Autodesk Inventor part; units mm, degrees
ref_plane "YZ Plane" through (0, 0, 0) normal (1, 0, 0) x (0, 1, 0)
ref_plane "XZ Plane" through (0, 0, 0) normal (0, 1, 0) x (-1, 0, 0)
ref_plane "XY Plane" through (0, 0, 0) normal (0, 0, 1) x (1, 0, 0)
sketch "スケッチ1" plane through (0, 0, 0) normal (0, 1, 0) x (-1, 0, 0)
  line L0 (7.5, -7.5) -> (-7.5, -7.5)
  line L1 (-7.5, -7.5) -> (-7.5, 7.5)
  line L2 (-7.5, 7.5) -> (7.5, 7.5)
  line L3 (7.5, 7.5) -> (7.5, -7.5)
  line L4 (7.5, -7.5) -> (-7.5, 7.5) construction
  line L5 (-7.5, -7.5) -> (7.5, 7.5) construction
  line L6 (6, -6) -> (-6, -6)
  line L7 (-6, -6) -> (-6, 6)
  line L8 (-6, 6) -> (6, 6)
  line L9 (6, 6) -> (6, -6)
  point P0 (0, 0)
  dimension "d0" = 15
  dimension "d1" = 15
  dimension "d2" = 1.5
extrude "押し出し1" add sketch "スケッチ1" along normal blind 88
sketch "スケッチ2" plane through (-7.5, 0, 7.5) normal (0, 0, 1) x (1, 0, 0)
  line L0 (7.5, 0) -> (7.5, 88) construction
  line L1 (0, 88) -> (15, 88)
  line L2 (0, 0) -> (0, 88)
  line L3 (0, 44) -> (15, 44) construction
  line L4 (15, 0) -> (15, 88)
sketch "スケッチ3" plane through (7.5, 0, 7.5) normal (1, 0, 0) x (0, 0, -1)
  line L0 (7.5, 0) -> (7.5, 88) construction
  line L1 (0, 88) -> (15, 88)
  line L2 (15, 0) -> (15, 88)
  line L3 (15, 44) -> (0, 44) construction
  line L4 (0, 0) -> (0, 88)
sketch "スケッチ4" plane through (-7.5, 0, 7.5) normal (0, 0, 1) x (1, 0, 0)
  line L0 (7.5, 0) -> (7.5, 88) construction
  circle A0 centre (7.5, 7.5) radius 1.5
  line L1 (0, 0) -> (15, 0)
  circle A1 centre (7.5, 68) radius 1.5
  line L2 (0, 88) -> (15, 88)
  dimension "d5" = 3
  dimension "d6" = 7.5
  dimension "d13" = 3
  dimension "d14" = 20
extrude "押し出し2" cut sketch "スケッチ4" against normal through all
sketch "スケッチ5" plane through (7.5, 0, 7.5) normal (1, 0, 0) x (0, 0, -1)
  circle A0 centre (7.5, 20) radius 1.5
  line L0 (7.5, 0) -> (7.5, 88) construction
  line L1 (0, 0) -> (15, 0)
  circle A1 centre (7.5, 80.5) radius 1.5
  line L2 (0, 88) -> (15, 88)
  dimension "d9" = 3
  dimension "d10" = 20
  dimension "d15" = 3
  dimension "d16" = 7.5
extrude "押し出し3" cut sketch "スケッチ5" against normal through all
sketch "スケッチ6" plane through (7.5, 0, 7.5) normal (1, 0, 0) x (0, 0, -1)
  circle A0 centre (7.5, 80.5) radius 1.5
  line L0 (0, 88) -> (15, 88)
  circle A1 centre (7.5, 20) radius 1.5
  line L1 (0, 0) -> (15, 0)
  point P0 (7.5, 0)
  dimension "d17" = 7.5
  dimension "d18" = 68
  dimension "d19" = 88
sketch "スケッチ7" plane through (-7.5, 0, 7.5) normal (0, 0, 1) x (1, 0, 0)
  circle A0 centre (7.5, 68) radius 1.5
  line L0 (0, 88) -> (15, 88)
  circle A1 centre (7.5, 7.5) radius 1.5
  point P0 (7.5, 0)
  dimension "d20" = 20
  dimension "d21" = 80.5
equation "\"d1\" = d0"
properties part number "omu_k_jo_11" material "アルミニウム 6061-AHC"
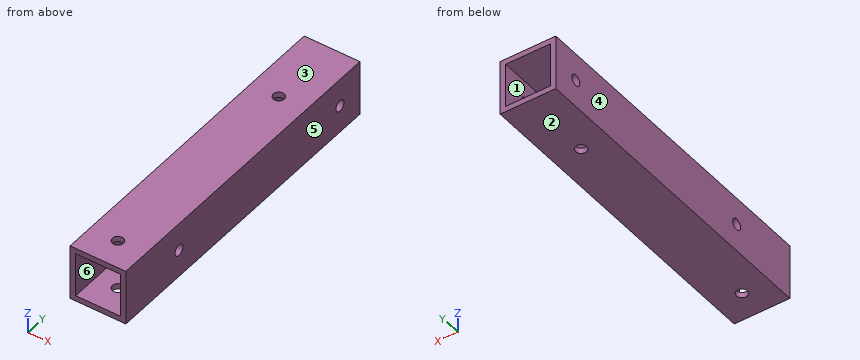
Design review of the part built by this model. Coordinates are the model's own, in mm. Face numbers are marked on the shaded views. A direction names the side the tool comes from. Round coordinates to 2 decimals unless told otherwise and drop trailing zeros. Write each loop counter-clockwise with the first axis right and the second up, starting at its lowest first coordinate (ties: lowest second). Pieces come first, ordered by that corner, then holes. Notation, with made-up numbers: (14, 51.5) - (61, 51.5) arc R16 ccw to (61, 63.5) - close; hole circle Ø1 at (-15, 24.25). An arc over 180 degrees is marked (long way). Return JSON: item names as keys, results as strings. Group by question number.
Item 1: We need section A-A on z = 0. Write out the cut boundary in (x, y).
Item 2: We need section C-C on y = 68. Write out the cut boundary in (x, z), and give its area (3 significant figures).
Item 3: Insertion check: P1, Ø2.5, axis at y = 80.5, z = 0, coming from the +X side. The pin has a flat end and moves straight along its axis. Give the tip position at first contact, or say it passes through.
Item 4: Machinability: for the marked faces 5 and 6, which of the approach directions +Z, -Z, +X, -X, +Y, -Y give a long, thin tool a straight path to every point of the face, cutting with its end or side? Answer none if there is none.
Item 5: The part is to be moulded in two halves that separate along Z. For the marked faces 1, 2, 3 and 4, say which applies: pulls with the +Z half, pulls with the -Z half, needs draft (parallel to the pull), parting line crosses it, or undercut.
Item 6: We need section D-D on x = -3.5. Write out the cut boundary in (y, z), and give its area (3 significant figures).
Item 7: For probe 1 along Y at (x, z) = (-6.4, 0); probe 2 along Z at (x, y) = (2.75, 51); probe 3 along Y at (x, z) = (0, -6.6), list the stretches that pass through material, from the lowest coordinate up. Write a range as [from, to].
Item 8: We need section B-B on x = 0. Write out the cut boundary in (y, z).
Model answer:
{
 "1": {"outline": "(-7.5, 0) - (-6, 0) - (-6, 18.5) - (-7.5, 18.5) - close; (-7.5, 21.5) - (-6, 21.5) - (-6, 79) - (-7.5, 79) - close; (-7.5, 82) - (-6, 82) - (-6, 88) - (-7.5, 88) - close; (6, 0) - (7.5, 0) - (7.5, 18.5) - (6, 18.5) - close; (6, 21.5) - (7.5, 21.5) - (7.5, 79) - (6, 79) - close; (6, 82) - (7.5, 82) - (7.5, 88) - (6, 88) - close"},
 "2": {"outline": "(-7.5, -7.5) - (-1.5, -7.5) - (-1.5, -6) - (-6, -6) - (-6, 6) - (-1.5, 6) - (-1.5, 7.5) - (-7.5, 7.5) - close; (1.5, -7.5) - (7.5, -7.5) - (7.5, 7.5) - (1.5, 7.5) - (1.5, 6) - (6, 6) - (6, -6) - (1.5, -6) - close", "area": "72.0 mm²"},
 "3": {"P1": "passes through"},
 "4": {"face 5": "+Z, -Z, +X, +Y, -Y", "face 6": "+Y, -Y"},
 "5": {"face 1": "undercut", "face 2": "pulls with the -Z half", "face 3": "pulls with the +Z half", "face 4": "needs draft"},
 "6": {"outline": "(0, -7.5) - (88, -7.5) - (88, -6) - (0, -6) - close; (0, 6) - (88, 6) - (88, 7.5) - (0, 7.5) - close", "area": "264 mm²"},
 "7": {"probe 1": "y = [0, 18.5], [21.5, 79], [82, 88]", "probe 2": "z = [-7.5, -6], [6, 7.5]", "probe 3": "y = [0, 6], [9, 66.5], [69.5, 88]"},
 "8": {"outline": "(0, -7.5) - (6, -7.5) - (6, -6) - (0, -6) - close; (0, 6) - (6, 6) - (6, 7.5) - (0, 7.5) - close; (9, -7.5) - (66.5, -7.5) - (66.5, -6) - (9, -6) - close; (9, 6) - (66.5, 6) - (66.5, 7.5) - (9, 7.5) - close; (69.5, -7.5) - (88, -7.5) - (88, -6) - (69.5, -6) - close; (69.5, 6) - (88, 6) - (88, 7.5) - (69.5, 7.5) - close"}
}
